```python
from build123d import *

# Parameters (mm, degrees)
EXTRUDE_1_DEPTH      = 22
EXTRUDE_1_DEPTH_BACK = 22
FILLET_1_R           = 3
EXTRUDE_2_DEPTH      = 6.5
EXTRUDE_2_DEPTH_BACK = 6.5
EXTRUDE_3_DEPTH      = 14
EXTRUDE_3_DEPTH_BACK = 14


with BuildPart() as part:
    # Эскиз1 → Бобышка-Вытянуть1 (new, two sides: drawn at the far end of the back side and taken through both)
    with BuildSketch(Plane.XY.offset(-EXTRUDE_1_DEPTH_BACK)):
        with BuildLine():
            Line((0, 43), (-2.105519461, 43))
            ThreePointArc((-2.105519461, 43), (-5.5, 21.5), (-2.105519461, 0))
            Line((-2.105519461, 0), (0, 0))
            ThreePointArc((0, 0), (-3.5, 21.5), (0, 43))
        make_face()
    extrude(amount=EXTRUDE_1_DEPTH + EXTRUDE_1_DEPTH_BACK)

    # Скругление1
    fillet_1_edges = [part.edges().sort_by_distance(p)[0] for p in [
        (-1.05275973, 0, -22),
        (-1.05275973, 43, -22),
        (-1.05275973, 0, 22),
        (-1.05275973, 43, 22),
    ]]
    fillet(fillet_1_edges, radius=FILLET_1_R)

    # Эскиз2 → Бобышка-Вытянуть2 (add, two sides: drawn at the far end of the back side and taken through both)
    with BuildSketch(Plane.XY.offset(-EXTRUDE_2_DEPTH_BACK)):
        Polygon((-2.105519461, 43), (-7.901074418, 41.447085729), (-8.237011137, 42), (-13.397493305, 38.939048547), (-13.13867426, 37.973122721), (-2.793911065, 40.744993665), align=None)
    extrude(amount=EXTRUDE_2_DEPTH + EXTRUDE_2_DEPTH_BACK)

    # Эскиз3 → Бобышка-Вытянуть3 (add, two sides: drawn at the far end of the back side and taken through both)
    with BuildSketch(Plane.XY.offset(-EXTRUDE_3_DEPTH_BACK)):
        Polygon((-2.105519461, 0), (-8, 0), (-8, -6), (-10, -6), (-10, 2), (-2.72022514, 2), align=None)
    extrude(amount=EXTRUDE_3_DEPTH + EXTRUDE_3_DEPTH_BACK)


solid = part.part
```
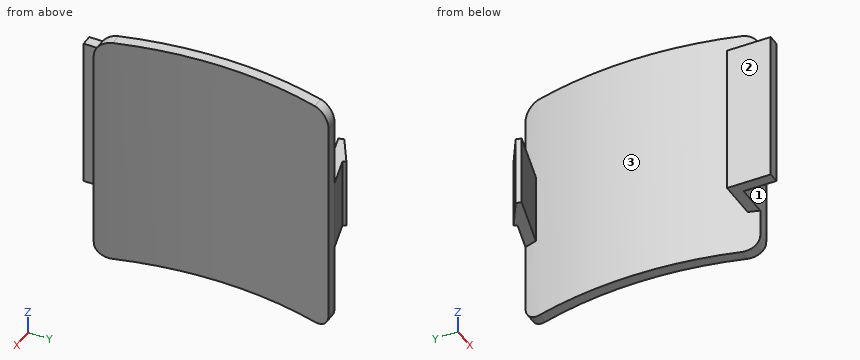
Build history of the part. All positions in model axes, mm. Face numbers are marked on the shaded views. Round coordinates to 2 decimals unless told otherwise and drop trailing zeros. Write each loop counter-clockwise with the first axis right and the second up, starting at its lowest first coordinate (ties: lowest second). Pieces come first, ordered by that corner, then holes.
1) Band-saw the part on C-C, the plane y = -3. List the corners of the cut face in (x, z).
2) Band-saw the part on D-D, the plane z = -3. List the corners of the cut face in (x, y) (1 decimal), and give its area (3 significant figures).
3) Mould opens along Y. For the marked faces 1, 2 and 3 say: +Y half, -Y half, draft (parallel to the pull), parting line (faces both ways), or undercut.
4) Pin check, flat tips, straight feed: pin 1 (5.5 mm diameter, centred on x = -6.5, y = 40.5, fed in from +Z); pin 2 (2 mm diameter, centred on x = -6.5, z = -3, fed in from +Y); pin 3 (8 mm diameter, centred on x = -11, y = 31, fed in from -Z); pin 4 (4 mm diameter, centred on x = -8, y = 41, fed in from -Z). Stop position of each tip, or through.
5) Band-saw the part on A-A, the plane z = -8. List the corners of the cut face in (x, y).
6) Drill centre lines: probe 1 along Y at (x, z) = (-7.75, -1); probe 2 along Z at (x, y) = (-9.5, 41); probe 3 along X at (y, z) = (26.5, -13.5). Where is each one in solid material? Low to high.
7) Band-saw the part on B-B, the plane x = -1.5. List the corners of the cut face in (y, z).
Ans:
1. outline: (-10, -14) - (-8, -14) - (-8, 14) - (-10, 14) - close
2. outline: (-13.4, 38.9) - (-13.1, 38) - (-2.8, 40.7) arc R69.8 ccw to (-2.7, 2) - (-10, 2) - (-10, -6) - (-8, -6) - (-8, 0) - (0, 0) arc R67.8 cw to (0, 43) - (-2.1, 43) - (-7.9, 41.4) - (-8.2, 42) - close
2. area: 136 mm2
3. face 1: -Y half
3. face 2: draft
3. face 3: undercut
4. pin 1: stops at z = 6.5
4. pin 2: stops at y = 42.09
4. pin 3: passes through
4. pin 4: stops at z = -6.5
5. outline: (-10, -6) - (-8, -6) - (-8, 0) - (0, 0) arc R67.79 cw to (0, 43) - (-2.11, 43) arc R69.79 ccw to (-2.72, 2) - (-10, 2) - close
6. probe 1: y = 0 to 2, 39.42 to 41.49
6. probe 2: z = -6.5 to 6.5
6. probe 3: x = -5.32 to -3.32
7. outline: (0, -19) arc R3 ccw to (3, -22) - (5.16, -22) - (5.16, 22) - (3, 22) arc R3 ccw to (0, 19) - close; (37.84, -22) - (40, -22) arc R3 ccw to (43, -19) - (43, 19) arc R3 ccw to (40, 22) - (37.84, 22) - close
